Part model, mm, in its own coordinate system. Give positions to 0.01 mm unless a question says otherwise; leave off trailing zeros. One line per question, with ' | ' between items.
Autodesk Fusion 360 part; units mm, degrees
sketch "Sketch1" plane through (0, 0, 0) normal (0, 1, 0) x (1, 0, 0)
  line L0 (9, -10) -> (-9, -10)
  line L1 (-10, -9) -> (-10, 9)
  line L2 (-9, 10) -> (9, 10)
  line L3 (10, 9) -> (10, -9)
  line L4 (10, -10) -> (-10, 10) construction
  line L5 (-10, -10) -> (10, 10) construction
  line L6 (4, -4) -> (-4, -4)
  line L7 (-4, -4) -> (-4, 4)
  line L8 (-4, 4) -> (4, 4)
  line L9 (4, 4) -> (4, -4)
  line L10 (4, -4) -> (-4, 4) construction
  line L11 (-4, -4) -> (4, 4) construction
  circle A0 centre (0, 0) radius 2
  line L12 (8.45, -8.45) -> (-8.45, -8.45)
  line L13 (-8.45, -8.45) -> (-8.45, 8.45)
  line L14 (-8.45, 8.45) -> (8.45, 8.45)
  line L15 (8.45, 8.45) -> (8.45, -8.45)
  line L16 (8.45, -8.45) -> (-8.45, 8.45) construction
  line L17 (-8.45, -8.45) -> (8.45, 8.45) construction
  line L18 (-9.452, -10.548) -> (10.548, 9.452) construction
  line L19 (-10.548, -9.452) -> (9.452, 10.548) construction
  line L20 (10.548, -9.452) -> (-9.452, 10.548) construction
  line L21 (9.452, -10.548) -> (-10.548, 9.452) construction
  line L22 (3.1, -10) -> (-3.1, -10) construction
  line L23 (-3.1, -10) -> (-3.1, 10) construction
  line L24 (-3.1, 10) -> (3.1, 10) construction
  line L25 (3.1, 10) -> (3.1, -10) construction
  line L26 (10, -3.1) -> (-10, -3.1) construction
  line L27 (-10, -3.1) -> (-10, 3.1) construction
  line L28 (-10, 3.1) -> (10, 3.1) construction
  line L29 (10, 3.1) -> (10, -3.1) construction
  line L30 (-3.1, -8.45) -> (-3.1, -10)
  line L31 (3.1, -8.45) -> (3.1, -10)
  line L32 (-8.45, -3.1) -> (-10, -3.1)
  line L33 (-8.45, 3.1) -> (-10, 3.1)
  line L34 (8.45, -3.1) -> (10, -3.1)
  line L35 (8.45, 3.1) -> (10, 3.1)
  line L36 (-3.1, 8.45) -> (-3.1, 10)
  line L37 (3.1, 8.45) -> (3.1, 10)
  line L38 (-4, 2.904) -> (-8.45, 7.354)
  line L39 (-2.904, 4) -> (-7.354, 8.45)
  line L40 (2.904, 4) -> (7.354, 8.45)
  line L41 (4, 2.904) -> (8.45, 7.354)
  line L42 (-4, -2.904) -> (-8.45, -7.354)
  line L43 (-2.904, -4) -> (-7.354, -8.45)
  line L44 (2.904, -4) -> (7.354, -8.45)
  line L45 (4, -2.904) -> (8.45, -7.354)
  line L46 (-10, -3.1) -> (-9.55, -3.1)
  line L47 (-9.55, -3.1) -> (-9.55, -3.6)
  line L48 (-9.55, -3.6) -> (-10, -3.6)
  line L49 (-10, -3.6) -> (-10, -3.1)
  line L50 (-10, 3.1) -> (-9.55, 3.1)
  line L51 (-9.55, 3.1) -> (-9.55, 3.6)
  line L52 (-9.55, 3.6) -> (-10, 3.6)
  line L53 (-10, 3.6) -> (-10, 3.1)
  line L54 (-3.1, -10) -> (-3.6, -10)
  line L55 (-3.6, -10) -> (-3.6, -9.55)
  line L56 (-3.6, -9.55) -> (-3.1, -9.55)
  line L57 (-3.1, -9.55) -> (-3.1, -10)
  line L58 (3.1, -10) -> (3.6, -10)
  line L59 (3.6, -10) -> (3.6, -9.55)
  line L60 (3.6, -9.55) -> (3.1, -9.55)
  line L61 (3.1, -9.55) -> (3.1, -10)
  line L62 (10, -3.1) -> (9.55, -3.1)
  line L63 (9.55, -3.1) -> (9.55, -3.6)
  line L64 (9.55, -3.6) -> (10, -3.6)
  line L65 (10, -3.6) -> (10, -3.1)
  line L66 (10, 3.1) -> (9.55, 3.1)
  line L67 (9.55, 3.1) -> (9.55, 3.6)
  line L68 (9.55, 3.6) -> (10, 3.6)
  line L69 (10, 3.6) -> (10, 3.1)
  line L70 (-3.1, 10) -> (-3.6, 10)
  line L71 (-3.6, 10) -> (-3.6, 9.55)
  line L72 (-3.6, 9.55) -> (-3.1, 9.55)
  line L73 (-3.1, 9.55) -> (-3.1, 10)
  line L74 (3.1, 10) -> (3.55, 10)
  line L75 (3.55, 10) -> (3.55, 9.5)
  line L76 (3.55, 9.5) -> (3.1, 9.5)
  line L77 (3.1, 9.5) -> (3.1, 10)
  arc A1 (-10, -9) -> (-9, -10) centre (-9, -9) ccw
  arc A2 (9, -10) -> (10, -9) centre (9, -9) ccw
  arc A3 (10, 9) -> (9, 10) centre (9, 9) ccw
  arc A4 (-9, 10) -> (-10, 9) centre (-9, 9) ccw
  arc A5 (29, -10) -> (30, -9) centre (29, -9) ccw
  line L78 (30, -3.1) -> (10, -3.1) construction
  line L79 (30, 9) -> (30, -9)
  line L80 (24, 4) -> (24, -4)
  line L81 (29.452, -10.548) -> (9.452, 9.452) construction
  line L82 (30, 3.1) -> (29.55, 3.1)
  line L83 (29, -10) -> (11, -10)
  line L84 (16, 4) -> (24, 4)
  line L85 (24, -4) -> (16, 4) construction
  line L86 (28.45, -8.45) -> (11.55, -8.45)
  circle A6 centre (20, 0) radius 2
  line L87 (10, -9) -> (10, 9)
  line L88 (10, -3.1) -> (10, 3.1) construction
  line L89 (16.9, 8.45) -> (16.9, 10)
  arc A7 (11, 10) -> (10, 9) centre (11, 9) ccw
  line L90 (17.096, -4) -> (12.646, -8.45)
  line L91 (16.9, -8.45) -> (16.9, -10)
  line L92 (16.4, -9.55) -> (16.9, -9.55)
  line L93 (10, -3.1) -> (10.45, -3.1)
  line L94 (10, 3.1) -> (10.45, 3.1)
  line L95 (10.45, 3.1) -> (10.45, 3.6)
  arc A8 (10, -9) -> (11, -10) centre (11, -9) ccw
  line L96 (10.45, -3.1) -> (10.45, -3.6)
  line L97 (16.9, -10) -> (16.9, 10) construction
  line L98 (10.45, -3.6) -> (10, -3.6)
  line L99 (29.55, 3.1) -> (29.55, 3.6)
  line L100 (16, -4) -> (16, 4)
  line L101 (23.1, -9.55) -> (23.1, -10)
  line L102 (28.45, -3.1) -> (30, -3.1)
  line L103 (30, -3.6) -> (30, -3.1)
  line L104 (22.904, -4) -> (27.354, -8.45)
  line L105 (22.904, 4) -> (27.354, 8.45)
  line L106 (23.1, 10) -> (23.1, -10) construction
  line L107 (16, -2.904) -> (11.55, -7.354)
  line L108 (16, 2.904) -> (11.55, 7.354)
  line L109 (16.4, 10) -> (16.4, 9.55)
  line L110 (17.096, 4) -> (12.646, 8.45)
  line L111 (10, -3.6) -> (10, -3.1)
  line L112 (16.9, -9.55) -> (16.9, -10)
  line L113 (23.1, 9.5) -> (23.1, 10)
  line L114 (23.6, -10) -> (23.6, -9.55)
  line L115 (10.45, 3.6) -> (10, 3.6)
  line L116 (24, -2.904) -> (28.45, -7.354)
  line L117 (23.55, 10) -> (23.55, 9.5)
  line L118 (10, 3.6) -> (10, 3.1)
  line L119 (11.55, 3.1) -> (10, 3.1)
  line L120 (11.55, -8.45) -> (11.55, 8.45)
  line L121 (23.1, -10) -> (23.6, -10)
  line L122 (11.55, -3.1) -> (10, -3.1)
  line L123 (29.55, -3.6) -> (30, -3.6)
  line L124 (16.4, 9.55) -> (16.9, 9.55)
  line L125 (23.1, 10) -> (23.55, 10)
  line L126 (16.9, 10) -> (16.4, 10)
  line L127 (16.4, -10) -> (16.4, -9.55)
  line L128 (10, 3.1) -> (30, 3.1) construction
  line L129 (24, 2.904) -> (28.45, 7.354)
  line L130 (23.55, 9.5) -> (23.1, 9.5)
  line L131 (23.1, -8.45) -> (23.1, -10)
  line L132 (16.9, 9.55) -> (16.9, 10)
  line L133 (23.1, -10) -> (16.9, -10) construction
  line L134 (30, -3.1) -> (29.55, -3.1)
  line L135 (30.548, -9.452) -> (10.548, 10.548) construction
  line L136 (23.6, -9.55) -> (23.1, -9.55)
  line L137 (29.55, -3.1) -> (29.55, -3.6)
  line L138 (16.9, 10) -> (23.1, 10) construction
  line L139 (30, 3.1) -> (30, -3.1) construction
  line L140 (23.1, 8.45) -> (23.1, 10)
  line L141 (16.9, -10) -> (16.4, -10)
  line L142 (24, -4) -> (16, -4)
  line L143 (16, -4) -> (24, 4) construction
  line L144 (10, -10) -> (30, 10) construction
  arc A9 (30, 9) -> (29, 10) centre (29, 9) ccw
  line L145 (11, 10) -> (29, 10)
  line L146 (28.45, 8.45) -> (28.45, -8.45)
  line L147 (9.452, -9.452) -> (29.452, 10.548) construction
  line L148 (30, 3.6) -> (30, 3.1)
  line L149 (28.45, 3.1) -> (30, 3.1)
  line L150 (11.55, -8.45) -> (28.45, 8.45) construction
  line L151 (11.55, 8.45) -> (28.45, 8.45)
  line L152 (29.55, 3.6) -> (30, 3.6)
  line L153 (30, -10) -> (10, 10) construction
  line L154 (28.45, -8.45) -> (11.55, 8.45) construction
  line L155 (10.548, -10.548) -> (30.548, 9.452) construction
  line L156 (9, -10) -> (11, -10)
  line L157 (9, 10) -> (11, 10)
  line L158 (8.45, -8.45) -> (11.55, -8.45)
  line L159 (8.45, 8.45) -> (11.55, 8.45)
  point P0 (20, 0)
  point P1 (20, 0)
  point P2 (20, 0)
  point P3 (20, 0)
  point P4 (20, 0)
  point P5 (20, 0)
  dimension "d1" = 20
  dimension "d2" = 20
  dimension "d3" = 8
  dimension "d4" = 8
  dimension "d5" = 4
  dimension "d6" = 16.9
  dimension "d7" = 16.9
  dimension "d8" = 0.775
  dimension "d9" = -0.775
  dimension "d10" = 0.775
  dimension "d11" = -0.775
  dimension "d12" = 6.2
  dimension "d13" = 20
  dimension "d14" = 20
  dimension "d15" = 6.2
  dimension "d16" = 1.55
  dimension "d17" = 1.55
  dimension "d18" = 1.55
  dimension "d19" = 1.55
  dimension "d20" = 1.55
  dimension "d21" = 1.55
  dimension "d22" = 1.55
  dimension "d23" = 1.55
  dimension "d24" = 0.45
  dimension "d25" = 0.5
  dimension "d26" = 0.45
  dimension "d27" = 0.5
  dimension "d28" = 0.5
  dimension "d29" = 0.45
  dimension "d30" = 0.5
  dimension "d31" = 0.45
  dimension "d32" = 0.45
  dimension "d33" = 0.5
  dimension "d34" = 0.45
  dimension "d35" = 0.5
  dimension "d36" = 0.5
  dimension "d37" = 0.45
  dimension "d38" = 0.45
  dimension "d39" = 0.5
  dimension "d40" = 1
  dimension "d41" = 1
  dimension "d42" = 1
  dimension "d43" = 1
  dimension "d48" = 0.775
  dimension "d49" = -0.775
  dimension "d50" = 0.775
  dimension "d51" = -0.775
  dimension "d52" = 20
  dimension "d53" = 20
  dimension "d54" = 8
  dimension "d55" = 8
  dimension "d56" = 4
  dimension "d57" = 16.9
  dimension "d58" = 16.9
  dimension "d59" = 6.2
  dimension "d60" = 20
  dimension "d61" = 20
  dimension "d62" = 6.2
  dimension "d63" = 1.55
  dimension "d64" = 1.55
  dimension "d65" = 1.55
  dimension "d66" = 1.55
  dimension "d67" = 1.55
  dimension "d68" = 1.55
  dimension "d69" = 1.55
  dimension "d70" = 1.55
  dimension "d71" = 0.45
  dimension "d72" = 0.5
  dimension "d73" = 0.45
  dimension "d74" = 0.5
  dimension "d75" = 0.5
  dimension "d76" = 0.45
  dimension "d77" = 0.5
  dimension "d78" = 0.45
  dimension "d79" = 0.45
  dimension "d80" = 0.5
  dimension "d81" = 0.45
  dimension "d82" = 0.5
  dimension "d83" = 0.5
  dimension "d84" = 0.45
  dimension "d85" = 0.45
  dimension "d86" = 0.5
  dimension "d87" = 1
  dimension "d88" = 1
  dimension "d89" = 1
  dimension "d90" = 1
extrude "Extrude2" add sketch "Sketch1" along normal blind 500 contours L0 L3 L12 L31 L59 L60 A2 L87 L158 | A2 A8 L156 | L3 L83 L86 L87 L91 L92 A8 L127 L158 | L6 L9 L12 L15 L44 L45 | L86 L90 L100 L107 L120 L142 | L0 L1 L12 L13 L30 L32 L47 L48 L55 L56 A1 | L6 L7 L8 L9 | L80 L84 L100 L142 | A5 L79 L83 L86 L102 L114 L123 L131 L136 L137 L146 | L6 L7 L12 L13 L42 L43 | L8 L9 L14 L15 L40 L41 | L80 L86 L104 L116 L142 L146 | L84 L100 L108 L110 L120 L151 | L2 L3 L14 L37 L75 L76 A3 L87 L159 | L3 L87 L89 A7 L109 L124 L145 L151 L159 | A3 A7 L157 | L7 L8 L13 L14 L38 L39 | L80 L84 L105 L129 L146 L151 | L1 L2 L13 L14 L33 L36 L51 L52 L71 L72 A4 | L79 L99 L117 L130 L140 A9 L145 L146 L149 L151 L152
equation "d6 = 20 mm - ( ( 1.55 * 2 ) * 1 mm )"
equation "d7 = 20 mm - ( ( 1.55 * 2 ) * 1 mm )"
equation "d8 = ( 1.55 / 2 ) * 1 mm"
equation "d9 = ( -1.55 / 2 ) * 1 mm"
equation "d10 = ( 1.55 / 2 ) * 1 mm"
equation "d11 = ( -1.55 / 2 ) * 1 mm"
equation "d48 = ( 1.55 / 2 ) * 1 mm"
equation "d49 = ( -1.55 / 2 ) * 1 mm"
equation "d50 = ( 1.55 / 2 ) * 1 mm"
equation "d51 = ( -1.55 / 2 ) * 1 mm"
equation "d57 = 20 mm - ( ( 1.55 * 2 ) * 1 mm )"
equation "d58 = 20 mm - ( ( 1.55 * 2 ) * 1 mm )"
1) Saw through at A-A (y = 140.5). State how many separate pieces and enclosed holes the cut face has, and give its area (3 significant figures).
Found:
separate pieces: 1 | enclosed holes: 3 | area: 296 mm2
2) Drill centre lines: line 1 (X direction, y = 324, z = 0); line 2 (X direction, y = 467.5, z = 8.5); line 3 (Z direction, x = 0, y = 228). Where is each one in solid material? Low to high.
Found:
line 1: -4 to -2, 2 to 4, 16 to 18, 22 to 24 | line 2: -10 to -3.1, 3.1 to 16.9, 23.1 to 30 | line 3: -4 to -2, 2 to 4
3) Pin check, flat tips, straight feed: P1, Ø0.5, axis at x = -9.5, y = 264.5, coming from the -Z side; P2, Ø3, axis at y = 178, z = -1, coming from the +X side; P3, Ø1, axis at y = 361, z = 0.5, coming from the -X side. Stop position of each tip, or through.
Found:
P1: z = -9.97 | P2: x = 24 | P3: x = -4
